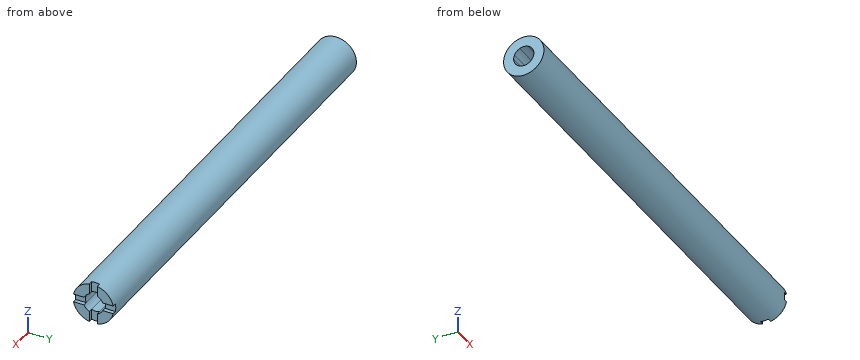
```python
from build123d import *

# Parameters (mm, degrees)
F0_W     = 52.451
F0_H     = 12.7
F0_W_2   = 207.899
F0_W_3   = 19.05
F3_DEPTH = 2.54
F4_DEPTH = 279.401


with BuildPart() as f1:
    # F0 (on Front) → F1 (revolve)
    with BuildSketch(Plane.XZ):
        with Locations((26.2255, 6.35)):
            Rectangle(F0_W, F0_H)
        with Locations((156.4005, 6.35)):
            Rectangle(F0_W_2, F0_H)
        with Locations((269.875, 6.35)):
            Rectangle(F0_W_3, F0_H)
    revolve(axis=Axis((26.2255, 0, 0), (-1, 0, 0)))

    # F2 (on face) → F3 (cut)
    with BuildSketch(Plane.YZ.offset(279.4)):
        with BuildLine():
            Line((2.54, 5.819871), (2.54, 12.443408))
            ThreePointArc((2.54, 12.443408), (0, 12.7), (-2.54, 12.443408))
            Line((-2.54, 12.443408), (-2.54, 5.819871))
            ThreePointArc((-2.54, 5.819871), (0, 6.35), (2.54, 5.819871))
        make_face()
        with BuildLine():
            Line((-5.819871, 2.54), (-12.443408, 2.54))
            ThreePointArc((-12.443408, 2.54), (-12.7, 0), (-12.443408, -2.54))
            Line((-12.443408, -2.54), (-5.819871, -2.54))
            ThreePointArc((-5.819871, -2.54), (-6.35, 0), (-5.819871, 2.54))
        make_face()
        with BuildLine():
            ThreePointArc((12.443408, -2.54), (12.635689, -1.276464), (12.7, 0))
            ThreePointArc((12.7, 0), (12.635689, 1.276464), (12.443408, 2.54))
            Line((12.443408, 2.54), (5.819871, 2.54))
            ThreePointArc((5.819871, 2.54), (6.216055, 1.297366), (6.35, 0))
            ThreePointArc((6.35, 0), (6.216055, -1.297366), (5.819871, -2.54))
            Line((5.819871, -2.54), (12.443408, -2.54))
        make_face()
        with BuildLine():
            ThreePointArc((-2.54, -12.443408), (0, -12.7), (2.54, -12.443408))
            Line((2.54, -12.443408), (2.54, -5.819871))
            ThreePointArc((2.54, -5.819871), (0, -6.35), (-2.54, -5.819871))
            Line((-2.54, -5.819871), (-2.54, -12.443408))
        make_face()
    extrude(amount=-F3_DEPTH, mode=Mode.SUBTRACT)

    # F2 (on face) → F4 (cut, through all)
    with BuildSketch(Plane.YZ.offset(279.4)):
        with BuildLine():
            ThreePointArc((6.35, 0), (6.216055, 1.297366), (5.819871, 2.54))
            ThreePointArc((5.819871, 2.54), (4.490128, 4.490128), (2.54, 5.819871))
            ThreePointArc((2.54, 5.819871), (0, 6.35), (-2.54, 5.819871))
            ThreePointArc((-2.54, 5.819871), (-4.490128, 4.490128), (-5.819871, 2.54))
            ThreePointArc((-5.819871, 2.54), (-6.35, 0), (-5.819871, -2.54))
            ThreePointArc((-5.819871, -2.54), (-4.490128, -4.490128), (-2.54, -5.819871))
            ThreePointArc((-2.54, -5.819871), (0, -6.35), (2.54, -5.819871))
            ThreePointArc((2.54, -5.819871), (4.490128, -4.490128), (5.819871, -2.54))
            ThreePointArc((5.819871, -2.54), (6.216055, -1.297366), (6.35, 0))
        make_face()
    extrude(amount=-F4_DEPTH, mode=Mode.SUBTRACT)


solid = f1.part
```
Source: CAD feature listing. Evaluate the final solid. Frame: model axes, mm. Coordinates: 2 decimals unless noted, no trailing zeros. Loops run counter-clockwise (first coordinate to the right, second up) from the corner with the lowest first, then second, coordinate; pieces in that order, holes last. Notation, with made-up numbers: M -11.75,9.5 L 30.25,9.5 A18 ccw 30.25,24.5 Z; hole C 53,7.5 d1. An arc over 180 degrees is marked long. Use a Markdown table: item, result. Add a question column.
Q1. Section query B-B, the plane x = 89. Return loops of the section in (y, z), and give its area (3 significant figures).
Q2. Material intervals for L1, parallel to Y at x = 257, z = -2.5; L2, parallel to Z at x = 79.5, y = -0.25; L3, parallel to Z at x = 133, y = -3.75, sorted ascending.
Q3. Section query A-A, the plane y = 0. Return loops of the section in (x, z).
Q4. First-contact query: pin 1 (2 mm diameter, centred on x = 278.5, z = 7.5, fed in from -Y); pin 2 (10 mm diameter, centred on y = 5, z = -6.5, fed in from -X); pin 3 (1.5 mm diameter, centred on y = 10, z = -0.5, fed in from +X); pin 4 (1.3 mm diameter, centred on x = 277.5, y = 10, fed in from -Z). Flat tips, straight axial feed; report the tip coordinate or a pass-through.
Result:
| question | item | result |
|---|---|---|
| 1 | outline | C 0,0 d25.4; hole M -5.82,-2.54 A6.35 ccw -2.54,-5.82 A6.35 ccw 2.54,-5.82 A6.35 ccw 5.82,-2.54 A6.35 ccw 6.35,0 A6.35 ccw 5.82,2.54 A6.35 ccw 2.54,5.82 A6.35 ccw -2.54,5.82 A6.35 ccw -5.82,2.54 A6.35 ccw Z |
| 1 | area | 380 mm2 |
| 2 | L1 | y = -12.45 to -5.84, 5.84 to 12.45 |
| 2 | L2 | z = -12.7 to -6.35, 6.35 to 12.7 |
| 2 | L3 | z = -12.13 to -5.12, 5.12 to 12.13 |
| 3 | outline | M 0,-12.7 L 276.86,-12.7 L 276.86,-6.35 L 0,-6.35 Z; M 0,6.35 L 276.86,6.35 L 276.86,12.7 L 0,12.7 Z |
| 4 | pin 1 | stops at y = -10.91 |
| 4 | pin 2 | stops at x = 0 |
| 4 | pin 3 | stops at x = 276.86 |
| 4 | pin 4 | stops at z = -8.59 |
